The model under review builds one solid part; all positions refer to its coordinate system, in mm. Give positions to 0.01 mm unless a question says otherwise; leave off trailing zeros. Order: outer loops, then holes, each group sorted by start corner. A loop starts at its lowest first (then second) coordinate and runs counter-clockwise, first axis right, second up.
```python
from build123d import *

# Parameters (mm, degrees)
SKETCH_1_W          = 100
SKETCH_1_H          = 30
EXTRUDE_1_DEPTH     = 200
SKETCH_3_R          = 1.5
CUT_EXTRUDE_1_DEPTH = 200


with BuildPart() as part:
    # 草圖1 → 填料-伸長1 (new body)
    with BuildSketch(Plane(origin=(0, 0, 0), x_dir=(1, 0, 0), z_dir=(0, 1, 0))):
        Rectangle(SKETCH_1_W, SKETCH_1_H)
    extrude(amount=EXTRUDE_1_DEPTH)

    # 草圖2 → 旋轉5 (revolve)
    with BuildSketch(Plane.XY.offset(15)):
        with BuildLine():
            Line((-15, 170), (15, 170))
            ThreePointArc((15, 170), (0, 185), (-15, 170))
        make_face()
    revolve(axis=Axis((-33.156754736, 170, 15), (1, 0, 0)))

    # 草圖3 → 除料-伸長1 (cut)
    with BuildSketch(Plane.ZY.offset(50)):
        with Locations((0, 40)):
            Circle(SKETCH_3_R)
    extrude(amount=-CUT_EXTRUDE_1_DEPTH, mode=Mode.SUBTRACT)


solid = part.part
```
Item 1: Take a section at D-D (z = 19). Give the boundary of the cut face in (x, y), and give its area (3 significant figures).
Values found:
outline: circle Ø28.91 at (0, 170)
area: 657 mm2
Item 2: Take a section at B-B (y = 178). Give the boundary of the cut face in (x, z), and give its area (3 significant figures).
Values found:
outline: (-50, -15) - (50, -15) - (50, 15) - (12.69, 15) arc R12.69 ccw to (-12.69, 15) - (-50, 15) - close
area: 3,250 mm2
Item 3: Take a section at A-A (x = -35). Give the boundary of the cut face in (y, z).
Values found:
outline: (0, -15) - (200, -15) - (200, 15) - (0, 15) - close; hole circle Ø3 at (40, 0)
Item 4: Take a section at C-C (x = -8). Give the boundary of the cut face in (y, z).
Values found:
outline: (0, -15) - (200, -15) - (200, 15) - (182.69, 15) arc R12.69 ccw to (157.31, 15) - (0, 15) - close; hole circle Ø3 at (40, 0)
Item 5: Clearance check with flat-ended pins moving along their axes: pin 1 Ø1 at (x, z) = (6, 17) entering from -Y; pin 2 Ø1 at (x, y) = (6.5, 60) entering from +Z. State where each tip first meets the part, or that it passes through.
Values found:
pin 1: stops at y = 156.18
pin 2: stops at z = 15
Item 6: For line 1 (Y direction, x = 28.5, z = 0); line 2 (Z direction, x = -45, y = 146.5); line 3 (Z direction, x = 42, y = 40.5), list the stretches that pass through material, from the lowest coordinate up.
Values found:
line 1: y = 0 to 38.5, 41.5 to 200
line 2: z = -15 to 15
line 3: z = -15 to -1.41, 1.41 to 15
